```python
from build123d import *

# Parameters (mm, degrees)
BOSS_EXTRUDE1_DEPTH            = 44
CUT_EXTRUDE1_DEPTH             = 35
CUT_EXTRUDE2_REACH             = 67.586
SKETCH2_R                      = 9.7
CBORE_FOR_M3_SHCS1_D           = 3.4
CBORE_FOR_M3_SHCS1_CBORE_D     = 6.5
CBORE_FOR_M3_SHCS1_CBORE_DEPTH = 3
CUT_EXTRUDE3_REACH             = 82.169
SKETCH6_R                      = 1.7
CUT_EXTRUDE4_DEPTH             = 2.8
CHAMFER1_SIZE                  = 1


with BuildPart() as part:
    # Sketch1 → Boss-Extrude1 (new body)
    with BuildSketch(Plane.XY):
        with BuildLine():
            Line((-9.452299133, -24.156520859), (-29.85, -24.156520859))
            ThreePointArc((-29.85, -24.156520859), (0, -38.4), (29.85, -24.156520859))
            Line((29.85, -24.156520859), (9.452299133, -24.156520859))
            ThreePointArc((9.452299133, -24.156520859), (0, -27.2), (-9.452299133, -24.156520859))
        make_face()
        with BuildLine():
            Line((29.85, 15.843479141), (-29.85, 15.843479141))
            Line((-29.85, 15.843479141), (-29.85, -24.156520859))
            Line((-29.85, -24.156520859), (-9.452299133, -24.156520859))
            ThreePointArc((-9.452299133, -24.156520859), (-7.392995132, 3.414701626), (16.2, -11))
            ThreePointArc((16.2, -11), (14.414701626, -18.392995132), (9.452299133, -24.156520859))
            Line((9.452299133, -24.156520859), (29.85, -24.156520859))
            Line((29.85, -24.156520859), (29.85, 15.843479141))
        make_face()
        with BuildLine():
            ThreePointArc((16.2, -11), (-7.392995132, 3.414701626), (-9.452299133, -24.156520859))
            Line((-9.452299133, -24.156520859), (9.452299133, -24.156520859))
            ThreePointArc((9.452299133, -24.156520859), (14.414701626, -18.392995132), (16.2, -11))
        make_face()
        with BuildLine():
            Line((9.452299133, -24.156520859), (-9.452299133, -24.156520859))
            ThreePointArc((-9.452299133, -24.156520859), (0, -27.2), (9.452299133, -24.156520859))
        make_face()
    extrude(amount=BOSS_EXTRUDE1_DEPTH)

    # Sketch1<3> → Cut-Extrude1 (cut)
    with BuildSketch(Plane.XY):
        with BuildLine():
            ThreePointArc((16.2, -11), (-7.392995132, 3.414701626), (-9.452299133, -24.156520859))
            Line((-9.452299133, -24.156520859), (9.452299133, -24.156520859))
            ThreePointArc((9.452299133, -24.156520859), (14.414701626, -18.392995132), (16.2, -11))
        make_face()
        with BuildLine():
            Line((9.452299133, -24.156520859), (-9.452299133, -24.156520859))
            ThreePointArc((-9.452299133, -24.156520859), (0, -27.2), (9.452299133, -24.156520859))
        make_face()
    extrude(amount=CUT_EXTRUDE1_DEPTH, mode=Mode.SUBTRACT)

    # Sketch2 → Cut-Extrude2 (cut, up to next)
    with BuildSketch(Plane.XY.offset(44), mode=Mode.PRIVATE) as cut_extrude2_sk1:
        with Locations((0, -11)):
            Circle(SKETCH2_R)
    cut_extrude2_tool1 = extrude(cut_extrude2_sk1.sketch, amount=-CUT_EXTRUDE2_REACH, mode=Mode.PRIVATE) & part.part
    add(cut_extrude2_tool1.solids().sort_by_distance((0, -11, 44))[0], mode=Mode.SUBTRACT)

    # CBORE for M3 SHCS1 (through all)
    with Locations(Plane.XY.offset(44)):
        with Locations((-12.21600407, -15.446261863), (12.21600407, -6.553738137), (4.446261863, -23.21600407), (-4.446261863, 1.21600407)):
            CounterBoreHole(CBORE_FOR_M3_SHCS1_D / 2, CBORE_FOR_M3_SHCS1_CBORE_D / 2, CBORE_FOR_M3_SHCS1_CBORE_DEPTH)

    # Sketch6 → Cut-Extrude3 (cut, up to next)
    with BuildSketch(Plane(origin=(0, -44.156520859, 0), x_dir=(-1, 0, 0), z_dir=(0, -1, 0)), mode=Mode.PRIVATE) as cut_extrude3_sk1:
        with Locations(Location((20.75, -12, 0), (0, 0, 180))):
            Circle(SKETCH6_R)
    cut_extrude3_tool1 = extrude(cut_extrude3_sk1.sketch, amount=-CUT_EXTRUDE3_REACH, mode=Mode.PRIVATE) & part.part
    # Sketch6 → Cut-Extrude3 (cut, up to next)
    with BuildSketch(Plane(origin=(0, -44.156520859, 0), x_dir=(-1, 0, 0), z_dir=(0, -1, 0)), mode=Mode.PRIVATE) as cut_extrude3_sk2:
        with Locations(Location((-20.75, -12, 0), (0, 0, 180))):
            Circle(SKETCH6_R)
    cut_extrude3_tool2 = extrude(cut_extrude3_sk2.sketch, amount=-CUT_EXTRUDE3_REACH, mode=Mode.PRIVATE) & part.part
    # Sketch6 → Cut-Extrude3 (cut, up to next)
    with BuildSketch(Plane(origin=(0, -44.156520859, 0), x_dir=(-1, 0, 0), z_dir=(0, -1, 0)), mode=Mode.PRIVATE) as cut_extrude3_sk3:
        with Locations(Location((20.75, -32, 0), (0, 0, 180))):
            Circle(SKETCH6_R)
    cut_extrude3_tool3 = extrude(cut_extrude3_sk3.sketch, amount=-CUT_EXTRUDE3_REACH, mode=Mode.PRIVATE) & part.part
    # Sketch6 → Cut-Extrude3 (cut, up to next)
    with BuildSketch(Plane(origin=(0, -44.156520859, 0), x_dir=(-1, 0, 0), z_dir=(0, -1, 0)), mode=Mode.PRIVATE) as cut_extrude3_sk4:
        with Locations(Location((-20.75, -32, 0), (0, 0, 180))):
            Circle(SKETCH6_R)
    cut_extrude3_tool4 = extrude(cut_extrude3_sk4.sketch, amount=-CUT_EXTRUDE3_REACH, mode=Mode.PRIVATE) & part.part
    add(cut_extrude3_tool1.solids().sort_by_distance((-20.75, -44.156521, 12))[0], mode=Mode.SUBTRACT)
    add(cut_extrude3_tool2.solids().sort_by_distance((20.75, -44.156521, 12))[0], mode=Mode.SUBTRACT)
    add(cut_extrude3_tool3.solids().sort_by_distance((-20.75, -44.156521, 32))[0], mode=Mode.SUBTRACT)
    add(cut_extrude3_tool4.solids().sort_by_distance((20.75, -44.156521, 32))[0], mode=Mode.SUBTRACT)

    # Sketch7 → Cut-Extrude4 (cut)
    with BuildSketch(Plane(origin=(0, -14.156520859, 0), x_dir=(1, 0, 0), z_dir=(0, 1, 0))):
        Polygon((-29.85, -14.9), (-29.85, -9.1), (-22.424315781, -9.1), (-24.098631561, -12), (-22.424315781, -14.9), align=None)
        Polygon((-24.098631561, -12), (-22.424315781, -14.9), (-22.424315781, -9.1), align=None)
        Polygon((-22.424315781, -14.9), (-22.424315781, -9.1), (-19.075684219, -9.1), (-17.401368439, -12), (-19.075684219, -14.9), align=None)
        Polygon((-29.85, -34.9), (-29.85, -29.1), (-22.424315781, -29.1), (-24.098631561, -32), (-22.424315781, -34.9), align=None)
        Polygon((-24.098631561, -32), (-22.424315781, -34.9), (-22.424315781, -29.1), align=None)
        Polygon((-22.424315781, -34.9), (-22.424315781, -29.1), (-19.075684219, -29.1), (-17.401368439, -32), (-19.075684219, -34.9), align=None)
        Polygon((22.424315781, -29.1), (22.424315781, -34.9), (19.075684219, -34.9), (17.401368439, -32), (19.075684219, -29.1), align=None)
        Polygon((29.85, -29.1), (29.85, -34.9), (22.424315781, -34.9), (24.098631561, -32), (22.424315781, -29.1), align=None)
        Polygon((24.098631561, -32), (22.424315781, -29.1), (22.424315781, -34.9), align=None)
        Polygon((24.098631561, -12), (22.424315781, -9.1), (29.85, -9.1), (29.85, -14.9), (22.424315781, -14.9), align=None)
        Polygon((22.424315781, -14.9), (24.098631561, -12), (22.424315781, -9.1), align=None)
        Polygon((22.424315781, -9.1), (19.075684219, -9.1), (17.401368439, -12), (19.075684219, -14.9), (22.424315781, -14.9), align=None)
    extrude(amount=-CUT_EXTRUDE4_DEPTH, mode=Mode.SUBTRACT)

    # Chamfer1
    chamfer1_edges = [part.edges().sort_by_distance(p)[0] for p in [
        (29.85, -16.956520859, 32),
        (29.85, -14.156520859, 32),
        (29.85, -15.556520859, 29.1),
        (29.85, -15.556520859, 34.9),
        (-29.85, -16.956520859, 32),
        (-29.85, -14.156520859, 32),
        (-29.85, -15.556520859, 34.9),
        (-29.85, -15.556520859, 29.1),
        (-29.85, -16.956520859, 12),
        (-29.85, -14.156520859, 12),
        (-29.85, -15.556520859, 14.9),
        (-29.85, -15.556520859, 9.1),
        (29.85, -16.956520859, 12),
        (29.85, -14.156520859, 12),
        (29.85, -15.556520859, 9.1),
        (29.85, -15.556520859, 14.9),
    ]]
    chamfer(chamfer1_edges, length=CHAMFER1_SIZE)


solid = part.part
```
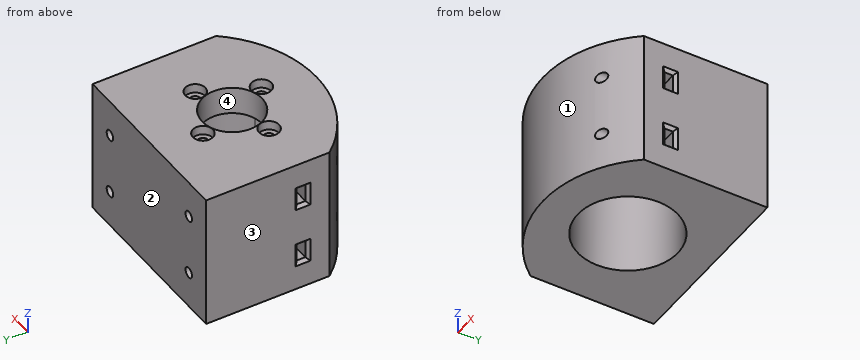
Can you work these out from the model? Positions are in its coordinate system, mm. Face numbers are marked on the shaded views. Coordinates: 2 decimals unless noted, no trailing zeros. Write each loop counter-clockwise with the first axis right and the second up, starting at its lowest first coordinate (ties: lowest second). Pieces come first, ordered by that corner, then holes. Notation, with made-up numbers: M 63.25,-6 L 104.25,-6 A22 cw 104.25,13 Z; hole C -28.75,49.5 d1. An arc over 180 degrees is marked long. Write item = value, one per line. Start each with the question number.
Q1. If we section it at C-C, the plane x = 2: Write out the boundary of the cut face in (y, z).
Q2. I'm going to push flat-ended pins straight in: pin 1 (1 mm diameter, centred on x = 9, z = 31, fed in from -Y); pin 2 (6 mm diameter, centred on x = 24, z = 7.5, fed in from -Y); pin 3 (7 mm diameter, centred on x = 5.5, y = -23, fed in from +Z); pin 4 (5.5 mm diameter, centred on x = -20.75, z = 12, fed in from -Y). Where does each tip first touch, or does it pass through?
Q3. Thinking about a two-plate mould opening in Y: for the marked faces 1, 2, 3 and 4, which applies, released by +Y, released by -Y, zero draft, split by the parting line, or undercut?
Q4. If we section it at B-B, the plane x = -20.75: Write out the boundary of the cut face in (y, z).
Q5. If I drill on L1, parallel to Z at x = 20.75, y = -26.5; L2, parallel to Z at x = -20, y = -3; L3, parallel to X at y = -10.5, z = 33, over which ranges is the centre line in solid material (lowest first)? Write a range as [from, to].
Q6. If we section it at A-A, the plane z = 3: Write out the boundary of the cut face in (x, y).
Q7. If we section it at D-D, the plane x = 20.5: Write out the boundary of the cut face in (y, z), then the cut area to 3 significant figures.
Check sheet entries:
q1.outline = M -38.35,0 L -27.08,0 L -27.08,35 L -20.49,35 L -20.49,44 L -21.08,44 L -21.08,41 L -25.36,41 L -25.36,44 L -38.35,44 Z; M -1.51,35 L 5.08,35 L 5.08,0 L 15.84,0 L 15.84,44 L -1.51,44 Z
q2.pin_1 = -37.45
q2.pin_2 = -32.15
q2.pin_3 = 44
q2.pin_4 = -33.92
q3.face_1 = released by -Y
q3.face_2 = released by +Y
q3.face_3 = zero draft
q3.face_4 = undercut
q4.outline = M -32.31,0 L 15.84,0 L 15.84,10.3 L -14.16,10.3 L -14.16,9.1 L -16.96,9.1 L -16.96,10.3 L -32.31,10.3 Z; M -32.31,13.7 L -16.96,13.7 L -16.96,14.9 L -14.16,14.9 L -14.16,13.7 L 15.84,13.7 L 15.84,30.3 L -14.16,30.3 L -14.16,29.1 L -16.96,29.1 L -16.96,30.3 L -32.31,30.3 Z; M -32.31,33.7 L -16.96,33.7 L -16.96,34.9 L -14.16,34.9 L -14.16,33.7 L 15.84,33.7 L 15.84,44 L -32.31,44 Z
q5.L1 = [0, 10.3], [13.7, 30.3], [33.7, 44]
q5.L2 = [0, 10.47], [13.53, 30.47], [33.53, 44]
q5.L3 = [-29.85, -22.12], [-19.38, -16.19], [16.19, 19.38], [22.12, 29.85]
q6.outline = M -29.85,-24.16 A38.4 ccw 29.85,-24.16 L 29.85,15.84 L -29.85,15.84 Z; hole C 0,-11 d32.4
q7.outline = M -32.47,0 L 15.84,0 L 15.84,10.32 L -14.16,10.32 L -14.16,9.1 L -16.96,9.1 L -16.96,10.32 L -32.47,10.32 Z; M -32.47,13.68 L -16.96,13.68 L -16.96,14.9 L -14.16,14.9 L -14.16,13.68 L 15.84,13.68 L 15.84,30.32 L -14.16,30.32 L -14.16,29.1 L -16.96,29.1 L -16.96,30.32 L -32.47,30.32 Z; M -32.47,33.68 L -16.96,33.68 L -16.96,34.9 L -14.16,34.9 L -14.16,33.68 L 15.84,33.68 L 15.84,44 L -32.47,44 Z
q7.area = 1,790 mm²
